Source: CAD feature listing. Evaluate the final solid. Frame: model axes, mm. Give positions to 0.01 mm unless a question says otherwise; leave off trailing zeros. Order: outer loops, then holes, each group sorted by start corner. A loop starts at its lowest first (then second) coordinate and runs counter-clockwise, first axis right, second up. Notation, with made-up numbers: (-28.75, 22.5) -> (14.25, 22.5) arc R13 ccw to (14.25, 37.5) -> close; hole circle Ø2 at (16.25, 31). An arc over 180 degrees is marked (long way). Use CSV: the item, a comma, the result in double quotes.
Autodesk Inventor part; units mm, degrees
ref_plane "YZ Plane" through (0, 0, 0) normal (1, 0, 0) x (0, 1, 0)
ref_plane "XZ Plane" through (0, 0, 0) normal (0, 1, 0) x (-1, 0, 0)
ref_plane "XY Plane" through (0, 0, 0) normal (0, 0, 1) x (1, 0, 0)
sketch "草图1" plane through (0, 0, 0) normal (0, 0, 1) x (1, 0, 0)
  line L0 (-4, 0) -> (4, 0)
  line L1 (-4, 0) -> (-4, 7.5)
  line L2 (4, 0) -> (4, 7.5)
  arc A0 (-1.5, 7.5) -> (1.5, 7.5) centre (0, 7.5) ccw
  line L3 (-4, 7.5) -> (-1.5, 7.5)
  line L4 (1.5, 7.5) -> (4, 7.5)
  line L5 (0, 7.5) -> (0, 0) construction
  dimension "长度" = 8
  dimension "高度" = 7.5
  dimension "d3" = 7.5
  dimension "孔径" = 3
  dimension "d5" = 7.5
extrude "拉伸1" add sketch "草图1" along normal blind 3
equation "\"d3\" = 高度"
equation "\"d5\" = 高度"
properties part number "顶杆支架" material "木材(桦木)"
1. Ray query, line 1 along X through (y, z) = (6.75, 0.65); line 2 along X through (y, z) = (7, 1.2); line 3 along Y through (x, z) = (0.25, 1.45). Return the intervals inside material, ascending.
Answer below:
line 1,"x = -4 to -1.3, 1.3 to 4"
line 2,"x = -4 to -1.41, 1.41 to 4"
line 3,"y = 0 to 6.02"
2. Section query A-A on z = 1.45. Return loops of the section in (x, y), plus the area to 3 significant figures.
Answer below:
outline,"(-4, 0) -> (4, 0) -> (4, 7.5) -> (1.5, 7.5) arc R1.5 cw to (-1.5, 7.5) -> (-4, 7.5) -> close"
area,"56.5 mm²"
3. Mould query, pull axis X, two halves, no side actions, for faces 1 (the flat face through (-4, 4, 1)), 2 (the flat face through (3, 7.5, 1)), 3 (the cylindrical face through (0, 6, 1)), 4 (the flat face through (4, 4, 1)). Classes: released by +X, released by -X, zero draft, split by the parting line, or undercut.
Answer below:
face 1,"released by -X"
face 2,"zero draft"
face 3,"undercut"
face 4,"released by +X"
4. Section query C-C on x = -1.25. Return loops of the section in (y, z).
Answer below:
outline,"(0, 0) -> (6.67, 0) -> (6.67, 3) -> (0, 3) -> close"
5. Section query B-B on x = 0. Return loops of the section in (y, z), plus the area to 3 significant figures.
Answer below:
outline,"(0, 0) -> (6, 0) -> (6, 3) -> (0, 3) -> close"
area,"18.0 mm²"
